Part print with two shaded views. Sizes in mm from the minimum x, y, z corner. A direction names the side the tool comes from. Give positions to 0.01 mm unless a question says otherwise; leave off trailing zeros. Write each loop counter-clockwise with the first axis right and the second up, starting at its lowest first coordinate (ties: lowest second). Pieces come first, ordered by that corner, then holes. Notation, with made-up numbers: (51.5, 63.25) - (76.5, 63.25) arc R8 cw to (76.5, 77.25) - close; hole circle Ø7 at (-37.5, -29.5). An arc over 180 degrees is marked (long way). Answer as a JSON object with one key per item and string values.
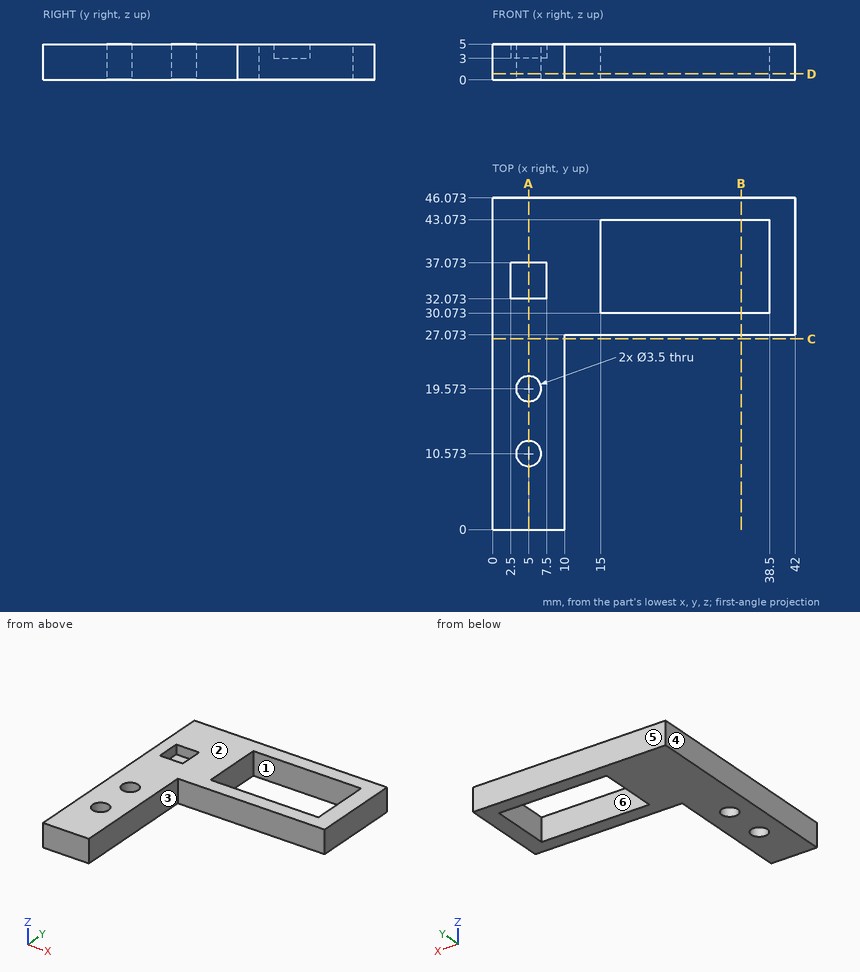
(1) Flat gauge pins, fed straight in: P1, Ø1.5, axis at x = 18, y = 30, coming from the -Z side; P2, Ø1.5, axis at x = 4, y = 35, coming from the +Z side; P3, Ø1.5, axis at y = 17, z = 2.5, coming from the +X side; P4, Ø1.5, axis at x = 25.5, z = 3.5, coming from the -Y side. Where does each tip first touch, or does it go through?
Answer key:
{"P1": "stops at z = 0", "P2": "stops at z = 3", "P3": "stops at x = 10", "P4": "stops at y = 27.07"}
(2) Saw through at D-D, the plane z = 0.85. Give the cut face in (x, y), and give its area (3 significant figures).
Answer key:
{"outline": "(0, 0) - (10, 0) - (10, 27.07) - (42, 27.07) - (42, 46.07) - (0, 46.07) - close; hole circle Ø3.5 at (5, 10.57); hole circle Ø3.5 at (5, 19.57); hole (15, 30.07) - (38.5, 30.07) - (38.5, 43.07) - (15, 43.07) - close", "area": "744 mm²"}
(3) Pull direction X, two halves, no side cores. Call the marked faces 4, 5 and 6: pulls with the +X half, pulls with the -X half, needs draft (parallel to the pull), parting line crosses it, or undercut.
Answer key:
{"face 4": "pulls with the -X half", "face 5": "needs draft", "face 6": "undercut"}
(4) Probe L1, parallel to Y at x = 5, z = 1.9; L2, parallel to Y at x = 36, z = 1.05; L3, parallel to Y at x = 5, z = 3.2. List the from-to ranges inside material, lowest first. Write a range as [from, to].
Answer key:
{"L1": "y = [0, 8.82], [12.32, 17.82], [21.32, 46.07]", "L2": "y = [27.07, 30.07], [43.07, 46.07]", "L3": "y = [0, 8.82], [12.32, 17.82], [21.32, 32.07], [37.07, 46.07]"}
(5) Saw through at C-C, the plane y = 26.5. Give the cut face in (x, z).
Answer key:
{"outline": "(0, 0) - (10, 0) - (10, 5) - (0, 5) - close"}
(6) Saw through at A-A, the plane x = 5. Give the cut face in (y, z).
Answer key:
{"outline": "(0, 0) - (8.82, 0) - (8.82, 5) - (0, 5) - close; (12.32, 0) - (17.82, 0) - (17.82, 5) - (12.32, 5) - close; (21.32, 0) - (46.07, 0) - (46.07, 5) - (37.07, 5) - (37.07, 3) - (32.07, 3) - (32.07, 5) - (21.32, 5) - close"}
(7) 3-axis set-ups, long thin cutter, end or side, ignore diameter. For the marked faces 1, 2 and 3: which of +Z, -Z, +X, -X, +Y, -Y reach the whole face in a straight line?
Answer key:
{"face 1": "+Z, -Z", "face 2": "+Z, +X, -X, +Y, -Y", "face 3": "+Z, -Z, +X, -Y"}
(8) Saw through at B-B, the plane x = 34.5. Give the cut face in (y, z), and give its area (3 significant figures).
Answer key:
{"outline": "(27.07, 0) - (30.07, 0) - (30.07, 5) - (27.07, 5) - close; (43.07, 0) - (46.07, 0) - (46.07, 5) - (43.07, 5) - close", "area": "30.0 mm²"}
